```python
from build123d import *

# Parameters (mm, degrees)
F1_DEPTH = 80
F4_DEPTH = 25
F6_DEPTH = 25
F7_DEPTH = 25
F9_DEPTH = 25
F10_R    = 7


with BuildPart() as f1:
    # F0 (on Right) → F1 (new body)
    with BuildSketch(Plane.YZ):
        Polygon((-73.535658, -7.88837), (-73.535658, -41.313667), (126.464342, -41.313667), (126.464342, 8.686333), (61.464342, 8.686333), (61.464342, 38.686333), (-8.535658, 38.686333), (-8.535658, 8.686333), (-43.535658, 8.686333), align=None)
    extrude(amount=F1_DEPTH)

    # F3 (on face) → F4 (cut)
    with BuildSketch(Plane(origin=(0, 0, 0), x_dir=(0, -1, 0), z_dir=(-1, 0, 0))):
        with BuildLine():
            Line((11.169364, -41.313667), (39.16015, -41.313667))
            ThreePointArc((39.16015, -41.313667), (25.164757, -27.672787), (11.169364, -41.313667))
        make_face()
    extrude(amount=-F4_DEPTH, mode=Mode.SUBTRACT)

    # F5 (on face) → F6 (cut)
    with BuildSketch(Plane(origin=(0, 0, 0), x_dir=(0, -1, 0), z_dir=(-1, 0, 0))):
        with BuildLine():
            Line((-85.647489, -41.313667), (-57.647489, -41.313667))
            ThreePointArc((-57.647489, -41.313667), (-71.647489, -27.313667), (-85.647489, -41.313667))
        make_face()
    extrude(amount=-F6_DEPTH, mode=Mode.SUBTRACT)

    # F2 (on face) → F7 (cut)
    with BuildSketch(Plane.YZ.offset(80)):
        with BuildLine():
            Line((-39.514016, -41.313667), (-11.518752, -41.313667))
            ThreePointArc((-11.518752, -41.313667), (-25.516384, -27.571131), (-39.514016, -41.313667))
        make_face()
    extrude(amount=-F7_DEPTH, mode=Mode.SUBTRACT)

    # F8 (on face) → F9 (cut)
    with BuildSketch(Plane.YZ.offset(80)):
        with BuildLine():
            Line((64.363025, -41.313667), (92.349545, -41.313667))
            ThreePointArc((92.349545, -41.313667), (78.356285, -26.879303), (64.363025, -41.313667))
        make_face()
    extrude(amount=-F9_DEPTH, mode=Mode.SUBTRACT)

    # F10
    f10_edges = [f1.edges().sort_by_distance(p)[0] for p in [
        (40, -8.535658, 38.686333),
        (40, -73.535658, -7.88837),
        (40, -43.535658, 8.686333),
    ]]
    fillet(f10_edges, radius=F10_R)


solid = f1.part
```
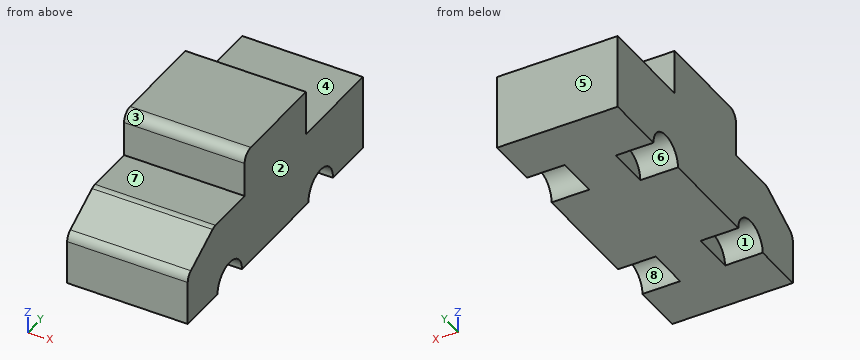
Input: part model. Units: mm. Frame: model coordinates. Face numbers are marked on the shaded views. A direction names the side the tool comes from. Coordinates: 2 decimals unless noted, no trailing zeros. Loops run counter-clockwise (first coordinate to the right, second up) from the corner with the lowest first, then second, coordinate; pieces in that order, holes last. Notation, with made-up numbers: M 33,37 L 84,37 A22 ccw 84,71 Z; hole C -31.5,-33 d2. An arc over 180 degrees is marked long. Answer in a Markdown table with one row per item.
1. Section B-B, the plane y = 81. Output: boundary loops of the cut face in (x, z).
Response:
| item | result |
|---|---|
| outline | M 0,-30.9 L 25,-30.9 L 25,-41.31 L 55,-41.31 L 55,-27.13 L 80,-27.13 L 80,8.69 L 0,8.69 Z |
2. Section C-C, the plane z = -32. Output: boundary loops of the cut face in (x, y).
Response:
| item | result |
|---|---|
| outline | M 0,-73.54 L 80,-73.54 L 80,-35.73 L 55,-35.73 L 55,-15.3 L 80,-15.3 L 80,67.53 L 55,67.53 L 55,89.18 L 80,89.18 L 80,126.46 L 0,126.46 L 0,82.1 L 25,82.1 L 25,61.19 L 0,61.19 L 0,-15.04 L 25,-15.04 L 25,-35.29 L 0,-35.29 Z |
3. Reachability of the marked faces 4, 5, 6, 7 and 8 from +Z, -Z, +X, -X, +Y, -Y: full face, straight path, thin tool, end or side. Return the list, or none.
Response:
| item | result |
|---|---|
| face 4 | +Z, +X, -X, +Y |
| face 5 | +Z, -Z, +X, -X, +Y |
| face 6 | -Z, -X |
| face 7 | +Z, +X, -X, -Y |
| face 8 | -Z, +X |
4. Section A-A, the plane x = 33. Output: boundary loops of the cut face in (y, z).
Response:
| item | result |
|---|---|
| outline | M -73.54,-41.31 L 126.46,-41.31 L 126.46,8.69 L 61.46,8.69 L 61.46,38.69 L -1.54,38.69 A7 ccw -8.54,31.69 L -8.54,8.69 L -41.73,8.69 A7 ccw -45.12,7.81 L -69.92,-5.89 A7 ccw -73.54,-12.02 Z |
5. Draft query along Y for the marked faces 1, 2 and 3. Return one class per face: pulls with the +Y half, pulls with the -Y half, needs draft (parallel to the pull), parting line crosses it, or undercut.
Response:
| item | result |
|---|---|
| face 1 | undercut |
| face 2 | needs draft |
| face 3 | pulls with the -Y half |
6. First-contact query: pin 1 (4.5 mm diameter, centred on y = 73.5, z = -37, fed in from +X); pin 2 (11.5 mm diameter, centred on x = 49.5, z = 16.5, fed in from -Y); pin 3 (7 mm diameter, centred on y = 71, z = -33.5, fed in from -X); pin 4 (8 mm diameter, centred on y = 33.5, z = -9.5, fed in from -X). Flat tips, straight axial feed; report the tip coordinate or a pass-through.
Response:
| item | result |
|---|---|
| pin 1 | stops at x = 55 |
| pin 2 | stops at y = -8.54 |
| pin 3 | stops at x = 25 |
| pin 4 | stops at x = 0 |
7. Material intervals for line 1 (Y direction, x = 77.5, z = 23); line 2 (Z direction, x = 29.5, y = -34); line 3 (Z direction, x = 12.5, y = 80.5), sorted ascending.
Response:
| item | result |
|---|---|
| line 1 | y = -8.54 to 61.46 |
| line 2 | z = -41.31 to 8.69 |
| line 3 | z = -30.47 to 8.69 |
8. Section D-D, the plane x = 13.5. Output: boundary loops of the cut face in (y, z).
Response:
| item | result |
|---|---|
| outline | M -73.54,-41.31 L -39.16,-41.31 A14 cw -11.17,-41.31 L 57.65,-41.31 A14 cw 85.65,-41.31 L 126.46,-41.31 L 126.46,8.69 L 61.46,8.69 L 61.46,38.69 L -1.54,38.69 A7 ccw -8.54,31.69 L -8.54,8.69 L -41.73,8.69 A7 ccw -45.12,7.81 L -69.92,-5.89 A7 ccw -73.54,-12.02 Z |
